Can you work these out from the drawing? Everything is in mm from the part's minimum corner. A direction names the side the tool comes from. Give positions to 0.01 mm unless a question says otherwise; leave off trailing zeros. Order: outer loops, then holes, each group sorted by start corner. A loop starts at its lowest first (then second) coordinate and runs counter-clockwise, first axis right, second up. Notation, with made-up numbers: M 8,49 L 13,49 A32 ccw 13,78 Z; hole C 73.5,3.5 d1. An arc over 180 degrees is marked long. Answer as a JSON object with one key per item and string values.
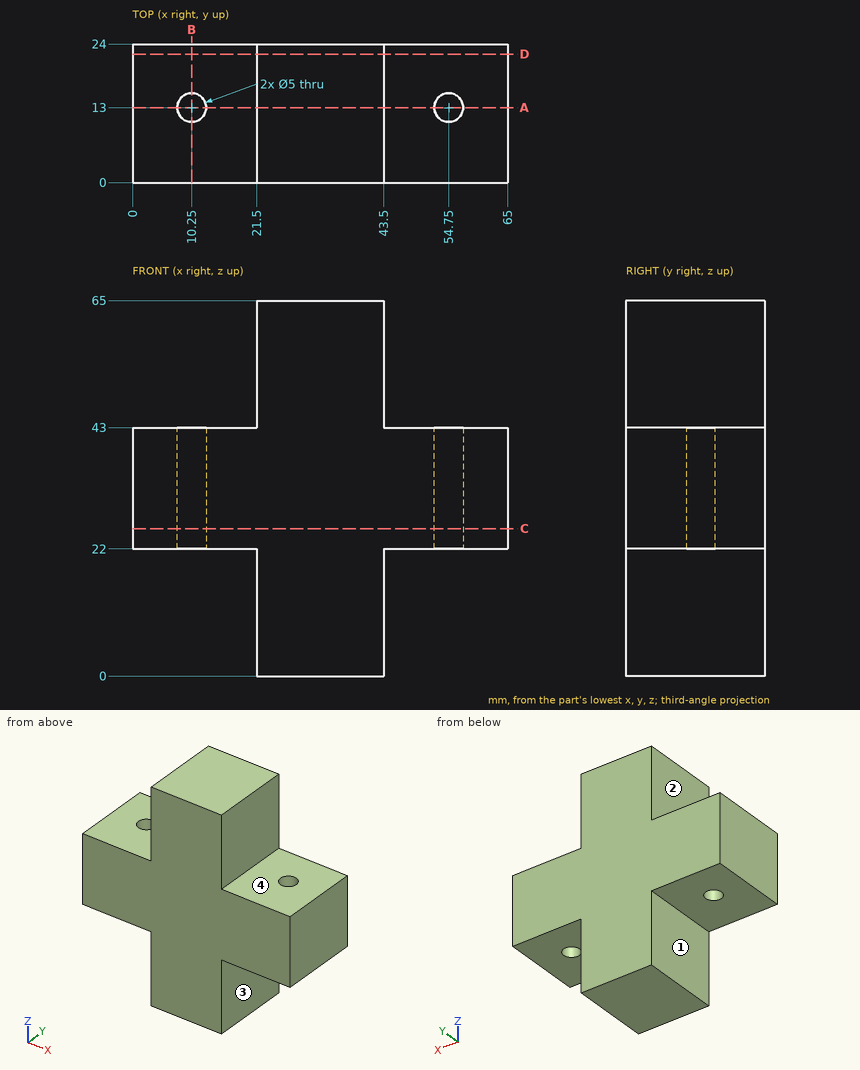
1) I want a section at B-B on x = 10.25. Write out the boundary of the cut face in (y, z), and give its area (3 significant figures).
Results found:
{"outline": "M 0,22 L 10.5,22 L 10.5,43 L 0,43 Z; M 15.5,22 L 24,22 L 24,43 L 15.5,43 Z", "area": "399 mm²"}
2) I'm going to push flat-ended pins straight in: pin 1 Ø6.5 at (x, y) = (54.75, 13) entering from -Z; pin 2 Ø1 at (y, z) = (21.5, 15) entering from -X; pin 3 Ø8 at (x, y) = (14.5, 3.5) entering from +Z; pin 4 Ø12 at (y, z) = (10, 43.5) entering from -X. Where does each tip first touch, or does it pass through?
Results found:
{"pin 1": "stops at z = 22", "pin 2": "stops at x = 21.5", "pin 3": "stops at z = 43", "pin 4": "stops at x = 0"}
3) I want a section at D-D on y = 22.25. Write out the boundary of the cut face in (x, z), and give its area (3 significant figures).
Results found:
{"outline": "M 0,22 L 21.5,22 L 21.5,0 L 43.5,0 L 43.5,22 L 65,22 L 65,43 L 43.5,43 L 43.5,65 L 21.5,65 L 21.5,43 L 0,43 Z", "area": "2,330 mm²"}
4) For the marked faces 1, 2, 3 and 4, which set-ups out of +Z, -Z, +X, -X, +Y, -Y let a thin tool reach every point of the face, with its end or its side?
Results found:
{"face 1": "-Z, -X, +Y, -Y", "face 2": "+Z, -X, +Y, -Y", "face 3": "-Z, +X, +Y, -Y", "face 4": "+Z, +X, +Y, -Y"}
5) I want a section at A-A on y = 13. Write out the boundary of the cut face in (x, z).
Results found:
{"outline": "M 0,22 L 7.75,22 L 7.75,43 L 0,43 Z; M 12.75,22 L 21.5,22 L 21.5,0 L 43.5,0 L 43.5,22 L 52.25,22 L 52.25,43 L 43.5,43 L 43.5,65 L 21.5,65 L 21.5,43 L 12.75,43 Z; M 57.25,22 L 65,22 L 65,43 L 57.25,43 Z"}
6) I want a section at C-C on z = 25.5. Write out the boundary of the cut face in (x, y).
Results found:
{"outline": "M 0,0 L 65,0 L 65,24 L 0,24 Z; hole C 10.25,13 d5; hole C 54.75,13 d5"}
7) I need wall thicknesses on L1, parallel to X at y = 13, z = 31; L2, parallel to Z at x = 13, y = 2.75; L3, parallel to X at y = 5.25, z = 45.5. Which ranges of each line are inside material? Lowest first, please.
Results found:
{"L1": "x = 0 to 7.75, 12.75 to 52.25, 57.25 to 65", "L2": "z = 22 to 43", "L3": "x = 21.5 to 43.5"}
